Can you work these out from the model? Positions are in its coordinate system, mm. A direction names the side the tool comes from. Coordinates: 2 decimals unless noted, no trailing zeros. Loops run counter-clockwise (first coordinate to the right, second up) from the corner with the lowest first, then second, coordinate; pieces in that order, holes last. Notation, with made-up numbers: M 20,53 L 33,53 A23 cw 33,69 Z; hole C -31,-34.5 d5. An arc over 180 degrees is marked long. Return JSON: item names as keys, results as strings. Group by question number.
```python
from build123d import *

# Parameters (mm, degrees)
HEADS_R                     = 6
HEAD_DEPTH                  = 1.5
TUBEENCAPSULATIONBODYS_R    = 3.5
TUBEENCAPSULATIONBODY_DEPTH = 6
TUBEACCESSS_R               = 3
TUBEACCESS_DEPTH            = 12.324751653
LOCKINGBODYS_R              = 4.9
LOCKINGBODYS_R_2            = 3
LOCKINGBODY_DEPTH           = 1
OPENCLAMPC_SIZE             = 0.5


with BuildPart() as part:
    # HeadS → Head (new body)
    with BuildSketch(Plane(origin=(0, 0, 0), x_dir=(1, 0, 0), z_dir=(0, 1, 0))):
        with Locations(Location((0, 0, 0), (0, 0, 270))):
            Circle(HEADS_R)
    extrude(amount=-HEAD_DEPTH)

    # TubeEncapsulationBodyS → TubeEncapsulationBody (add)
    with BuildSketch(Plane(origin=(0, 0, 0), x_dir=(-1, 0, 0), z_dir=(0, -1, 0))):
        with Locations(Location((0, 0, 0), (0, 0, 90))):
            Circle(TUBEENCAPSULATIONBODYS_R)
    extrude(amount=-TUBEENCAPSULATIONBODY_DEPTH)

    # TubeAccessS → TubeAccess (cut, through all)
    with BuildSketch(Plane(origin=(0, -1.5, 0), x_dir=(1, 0, 0), z_dir=(0, 1, 0))):
        with Locations(Location((0, 0, 0), (0, 0, 270))):
            Circle(TUBEACCESSS_R)
    extrude(amount=TUBEACCESS_DEPTH, mode=Mode.SUBTRACT)

    # LockingBodyS → LockingBody (add)
    with BuildSketch(Plane(origin=(0, 6, 0), x_dir=(1, 0, 0), z_dir=(0, 1, 0))):
        with Locations(Location((0, 0, 0), (0, 0, 270))):
            Circle(LOCKINGBODYS_R)
        with Locations(Location((0, 0, 0), (0, 0, 270))):
            Circle(LOCKINGBODYS_R_2, mode=Mode.SUBTRACT)
    extrude(amount=LOCKINGBODY_DEPTH)

    # OpenClampC
    openclampc_edges = [part.edges().sort_by_distance(p)[0] for p in [
        (0, 7, -4.9),
    ]]
    chamfer(openclampc_edges, length=OPENCLAMPC_SIZE)


solid = part.part
```
1) Suppose I cut it at C-C, the plane y = 2.25. List the corners of the cut face in (x, z) for me.
2) If we mould it in two halves opening along Y, with no side actions, what happens to faces 1 (the face through (3, -1.5, 1)), 2 (the face through (-3.2, 6, 2.1)), 3 (the face through (1.802, -0.74, 5.723))? For each: +Y half, -Y half, draft (parallel to the pull), parting line (faces both ways), or undercut.
3) For pin 1 (3 mm diameter, centred on y = 2.5, z = -3.5, fed in from +X); pin 2 (5 mm diameter, centred on y = 5.5, z = -3.5, fed in from -X); pin 3 (1.5 mm diameter, centred on y = 2.5, z = -3.5, fed in from -X), each with a flat end and sliding along its axis, tell me the tip position at first contact or that it passes through.
4) For faces 4 (the face through (-3.417, 2.958, 0.759)), 5 (the face through (1.472, 6.246, 4.674)), 6 (the face through (0.9, 2.69, 2.86)), which set-ups out of +Z, -Z, +X, -X, +Y, -Y let a thin tool reach every point of the face, with its end or its side?
5) Suppose I cut it at B-B, the plane z = 0. List the corners of the cut face in (x, y) for me.
6) If I drill on line 1 (Y direction, x = 0.75, z = -3.5); line 2 (X direction, y = 3.5, z = 0); line 3 (Z direction, x = 2.25, y = 2.75), over which ranges is the centre line in solid material (lowest first)? Write a range as from..to.
7) Suppose I cut it at A-A, the plane x = 0. List the corners of the cut face in (y, z) for me, then the cut area to 4 significant figures.
Returned:
{
 "1": {"outline": "C 0,0 d7; hole C 0,0 d6"},
 "2": {"face 1": "-Y half", "face 2": "undercut", "face 3": "draft"},
 "3": {"pin 1": "stops at x = 2.87", "pin 2": "stops at x = -4.79", "pin 3": "stops at x = -2.17"},
 "4": {"face 4": "none", "face 5": "+Y", "face 6": "+Y, -Y"},
 "5": {"outline": "M -6,-1.5 L -3,-1.5 L -3,7 L -4.4,7 L -4.9,6.5 L -4.9,6 L -3.5,6 L -3.5,0 L -6,0 Z; M 3,-1.5 L 6,-1.5 L 6,0 L 3.5,0 L 3.5,6 L 4.9,6 L 4.9,6.5 L 4.4,7 L 3,7 Z"},
 "6": {"line 1": "y = -1.5..0, 6..7", "line 2": "x = -3.5..-3, 3..3.5", "line 3": "z = -2.68..-1.98, 1.98..2.68"},
 "7": {"outline": "M -1.5,-6 L 0,-6 L 0,-3.5 L 6,-3.5 L 6,-4.9 L 6.5,-4.9 L 7,-4.4 L 7,-3 L -1.5,-3 Z; M -1.5,3 L 7,3 L 7,4.4 L 6.5,4.9 L 6,4.9 L 6,3.5 L 0,3.5 L 0,6 L -1.5,6 Z", "area": "18.55 mm²"}
}
